from build123d import *

# Parameters (mm, degrees)
SKETCH2_W           = 19.5
SKETCH2_H           = 19.5
BOSS_EXTRUDE1_DEPTH = 6
SKETCH3_R           = 5
BOSS_EXTRUDE2_DEPTH = 78
CHAMFER1_SIZE       = 1


with BuildPart() as part:
    # Sketch2 → Boss-Extrude1 (new body)
    with BuildSketch(Plane.XY):
        Rectangle(SKETCH2_W, SKETCH2_H)
    extrude(amount=BOSS_EXTRUDE1_DEPTH)

    # Sketch3 → Boss-Extrude2 (add)
    with BuildSketch(Plane.XY.offset(6)):
        Circle(SKETCH3_R)
    extrude(amount=BOSS_EXTRUDE2_DEPTH)

    # Chamfer1
    chamfer1_edges = [part.edges().sort_by_distance(p)[0] for p in [
        (-5, 0, 84),
    ]]
    chamfer(chamfer1_edges, length=CHAMFER1_SIZE)

    # Sketch4 → Cut-Revolve1 (revolve, cut)
    with BuildSketch(Plane(origin=(0, 0, 0), x_dir=(1, 0, 0), z_dir=(0, 1, 0))):
        with BuildLine():
            Line((0, 8.673011737), (0, 0))
            ThreePointArc((0, 0), (17.67766953, -7.32233047), (25, -25))
            Line((25, -25), (33.673011737, -25))
            ThreePointArc((33.673011737, -25), (23.810414942, -1.189585058), (0, 8.673011737))
        make_face()
    revolve(axis=Axis((0, 0, 0), (0, 0, 1)), mode=Mode.SUBTRACT)


solid = part.part
The listing builds one solid part. Answer for the finished solid, in the listing's coordinates (mm). A direction names the side the tool comes from. Round coordinates to 2 decimals unless told otherwise and drop trailing zeros. Order: outer loops, then holes, each group sorted by start corner. A loop starts at its lowest first (then second) coordinate and runs counter-clockwise, first axis right, second up. Notation, with made-up numbers: M 58.5,48.5 L 96.5,48.5 A35 cw 96.5,87.5 Z; hole C 53.25,7.5 d11. An arc over 180 degrees is marked long. Answer in a Markdown table with one row per item. Add a question column.
1) The part is cut by section C-C on z = 60.5. Determine the outline of the cut face in (x, y).
2) The part is cut by section D-D on y = 8.5. Determine the outline of the cut face in (x, z), plus the area to 3 significant figures.
3) Which of the six approach directions +Z, -Z, +X, -X, +Y, -Y give full straight-line access (tool end or side, diameter ignored) to faces 1 (the face through (-4, 4, 6)), 2 (the face through (9.75, 0, 4))?
4) Consider line 1 along Z through (x, y) = (-1.5, 2); line 2 along Z through (x, y) = (-8.5, -8.5); line 3 along Y through (x, z) = (-3.75, 17). Determine where each line is inside the solid, lowest interval first. Write a range as from..to.
5) The part is cut by section A-A on x = 0. Determine the outline of the cut face in (y, z).
6) Flat-ended cylindrical pins translate along their axes: pin 1 Ø3 at (y, z) = (3.5, 39) entering from +X; pin 2 Ø5 at (x, y) = (5.5, 0.5) entering from +Z; pin 3 Ø1.5 at (y, z) = (-5, 69.5) entering from +X; pin 4 Ø1 at (x, y) = (5.5, -1) entering from -Z. Find the tip coordinate at first contact, or state that the pin passes through.
Findings below:
| question | item | result |
|---|---|---|
| 1 | outline | C 0,0 d10 |
| 2 | outline | M -9.75,3.61 A23.51 ccw 9.75,3.61 L 9.75,6 L -9.75,6 Z |
| 2 | area | 74.5 mm² |
| 3 | face 1 | +Z |
| 3 | face 2 | +Z, -Z, +X, +Y, -Y |
| 4 | line 1 | z = 0.13..84 |
| 4 | line 2 | z = 3.08..6 |
| 4 | line 3 | y = -3.31..3.31 |
| 5 | outline | M -9.75,1.98 A25 ccw 9.75,1.98 L 9.75,6 L 5,6 L 5,83 L 4,84 L -4,84 L -5,83 L -5,6 L -9.75,6 Z |
| 6 | pin 1 | stops at x = 4.58 |
| 6 | pin 2 | stops at z = 84 |
| 6 | pin 3 | stops at x = 2.63 |
| 6 | pin 4 | stops at z = 0.52 |
